The drawing under review shows one solid part. Ordinate dimensions are in mm from its lowest x, y, z. Coordinates: 2 decimals unless noted, no trailing zeros. Write each loop counter-clockwise with the first axis right and the second up, starting at its lowest first coordinate (ties: lowest second). Pieces come first, ordered by that corner, then holes.
1) Add section C-C, the plane x = 52.5. State the section outline as (y, z) points, then the cut area to 3 significant figures.
2) For P1, Ø9, axis at x = 55, z = 55, coming from the -Y side; P2, Ø1.5, axis at x = 87, y = 1.5, coming from the -Z side; P3, Ø1.5, axis at x = 71, y = 2.5, coming from the -Z side; P4, Ø1.5, axis at x = 70.5, y = 2, coming from the -Z side (1 decimal), all flat-tipped, find the tip position at first contact; note any pin that passes through.
3) For line 1 (X direction, y = 1, z = 55); line 2 (X direction, y = 1.5, z = 45.5) (1 decimal); line 3 (X direction, y = 1.75, z = 32.5), list the stretches that pass through material, from the lowest coordinate up.
4) Add section A-A, the plane x = 80. State the section outline as (y, z) points, then the cut area to 3 significant figures.
5) Add section B-B, the plane y = 0.7. Give the number of separate pieces and of enclosed holes in the cut face, then the cut area to 3 significant figures.
6) Add section D-D, the plane z = 67.5. State the section outline as (x, y) points, then the cut area to 3 significant figures.
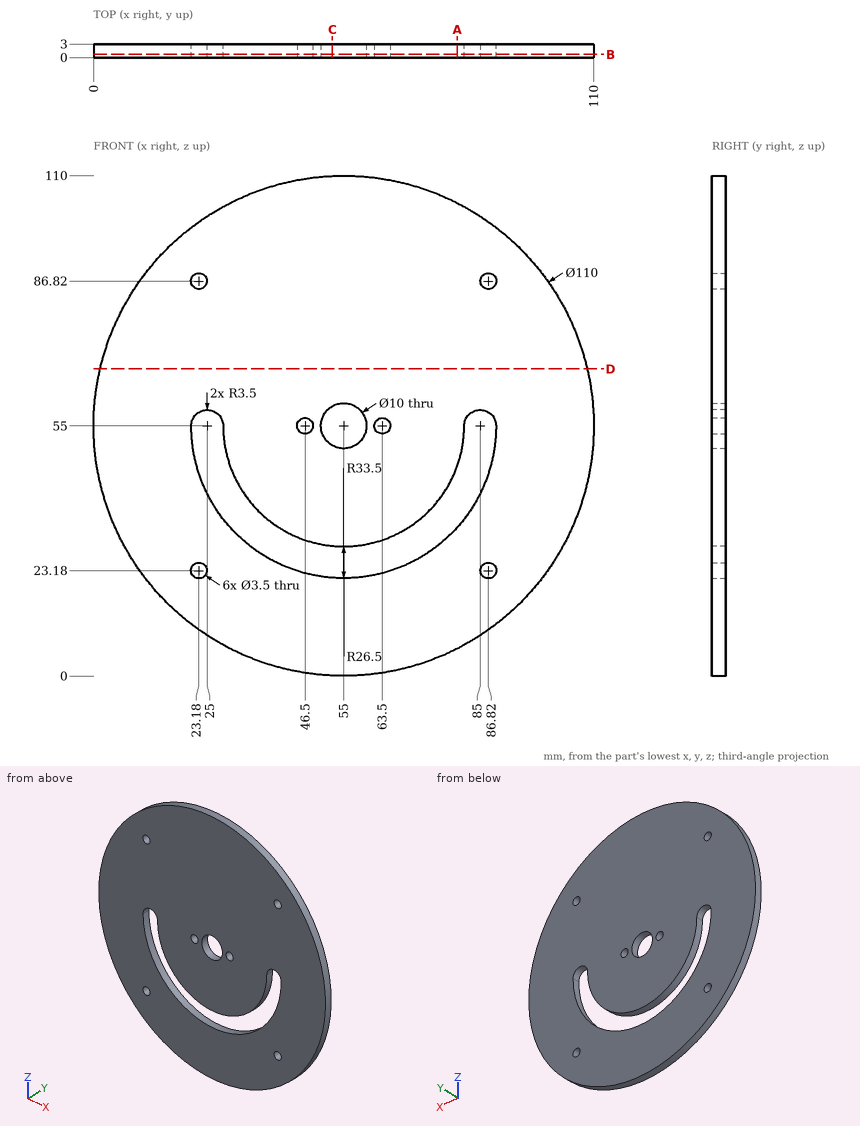
Geometry results:
1. outline: (0, 0.06) - (3, 0.06) - (3, 21.59) - (0, 21.59) - close; (0, 28.62) - (3, 28.62) - (3, 50.67) - (0, 50.67) - close; (0, 59.33) - (3, 59.33) - (3, 109.94) - (0, 109.94) - close
1. area: 283 mm2
2. P1: passes through
2. P2: stops at z = 9.74
2. P3: stops at z = 2.16
2. P4: stops at z = 2
3. line 1: x = 0 to 21.5, 28.5 to 44.75, 48.25 to 50, 60 to 61.75, 65.25 to 81.5, 88.5 to 110
3. line 2: x = 0.8 to 22.9, 30.3 to 79.7, 87.1 to 109.2
3. line 3: x = 4.81 to 30.18, 41 to 69, 79.82 to 105.19
4. outline: (0, 6.01) - (3, 6.01) - (3, 32.7) - (0, 32.7) - close; (0, 46.21) - (3, 46.21) - (3, 103.99) - (0, 103.99) - close
4. area: 253 mm2
5. separate pieces: 1
5. enclosed holes: 8
5. area: 8,670 mm2
6. outline: (1.44, 0) - (108.56, 0) - (108.56, 3) - (1.44, 3) - close
6. area: 321 mm2
